Input: part model. Units: mm. Frame: model coordinates. A direction names the side the tool comes from. Coordinates: 2 decimals unless noted, no trailing zeros. Write each loop counter-clockwise with the first axis right and the second up, starting at its lowest first coordinate (ties: lowest second). Pieces come first, ordered by that corner, then holes. Notation, with made-up numbers: M 26,57 L 43,57 A8 cw 43,66 Z; hole C 45,30.5 d6. An arc over 180 degrees is marked long. Write each question's results on one line, items separated by ' | '. Start each with the question number.
1. Section query A-A, the plane z = 38.1. Output: boundary loops of the cut face in (x, y), and give its area (4 significant figures).
2. Section query B-B, the plane x = 31.75. Output: boundary loops of the cut face in (y, z).
3. Section query D-D, the plane x = 11. Output: boundary loops of the cut face in (y, z).
4. Pull-direction query (Z, two-part tool) for faces 1 (the flat face through (31, 3, 101.6)), 2 (the flat face through (0, 5, 40)), 3 (the flat face through (31, 16, 0)), 4 (the cylindrical face through (32.68, 3.219, 45.183)); classes: +Z half, -Z half, draft (parallel to the pull), parting line (faces both ways), or undercut.
5. Ray query, probe 1 along X at (y, z) = (3, 38); probe 2 along Y at (x, z) = (6, 36); probe 3 along Z at (x, y) = (37, 3.5). Return the intervals inside material, ascending.
6. Set-up query: faces 5 (the flat face through (31, 19, 6.35)), 6 (the flat face through (31, 0, 52)). Return all of +Z, -Z, +X, -X, +Y, -Y with unobstructed straight access to the full face (end or side cutting, diameter ignored); none if empty.
7. First-contact query: pin 1 (19 mm diameter, centred on x = 38.5, z = 46, fed in from +Y); pin 2 (7.5 mm diameter, centred on x = 44.5, y = 21, fed in from +Z). Flat tips, straight axial feed; report the tip coordinate or a pass-through.
8. Section query C-C, the plane y = 4. Output: boundary loops of the cut face in (x, z), and give its area (3 significant figures).
```python
from build123d import *

# Parameters (mm, degrees)
F1_DEPTH = 63.5
F3_D     = 14.2875


with BuildPart() as f1:
    # F0 (on Right) → F1 (new body)
    with BuildSketch(Plane.YZ):
        Polygon((0, 101.6), (0, 0), (31.75, 0), (31.75, 6.35), (6.35, 6.35), (6.35, 101.6), align=None)
    extrude(amount=F1_DEPTH)

    # F3 (through all)
    with Locations(Plane.XZ):
        with Locations((31.75, 38.1)):
            Hole(F3_D / 2)


solid = f1.part
```
Answer:
1) outline: M 0,0 L 24.61,0 L 24.61,6.35 L 0,6.35 Z; M 38.89,0 L 63.5,0 L 63.5,6.35 L 38.89,6.35 Z | area: 312.5 mm^2
2) outline: M 0,0 L 31.75,0 L 31.75,6.35 L 6.35,6.35 L 6.35,30.96 L 0,30.96 Z; M 0,45.24 L 6.35,45.24 L 6.35,101.6 L 0,101.6 Z
3) outline: M 0,0 L 31.75,0 L 31.75,6.35 L 6.35,6.35 L 6.35,101.6 L 0,101.6 Z
4) face 1: +Z half | face 2: draft | face 3: -Z half | face 4: undercut
5) probe 1: 0 to 24.61, 38.89 to 63.5 | probe 2: 0 to 6.35 | probe 3: 0 to 33.26, 42.94 to 101.6
6) face 5: +Z, +X, -X, +Y | face 6: +Z, -Z, +X, -X, -Y
7) pin 1: y = 6.35 | pin 2: z = 6.35
8) outline: M 0,0 L 63.5,0 L 63.5,101.6 L 0,101.6 Z; hole C 31.75,38.1 d14.29 | area: 6,290 mm^2
